Can you work these out from the drawing? Everything is in mm from the part's minimum corner. Give positions to 0.01 mm unless a question says otherwise; leave off trailing zeros. Write each loop counter-clockwise with the first axis right and the second up, starting at its lowest first coordinate (ties: lowest second). Pieces come first, ordered by that corner, then holes. Notation, with made-up numbers: (16, 7.5) - (38, 7.5) arc R18 ccw to (38, 26.5) - close; hole circle Ø4 at (-23.5, 9). An arc over 180 degrees is marked (long way). Use a Markdown table: item, result.
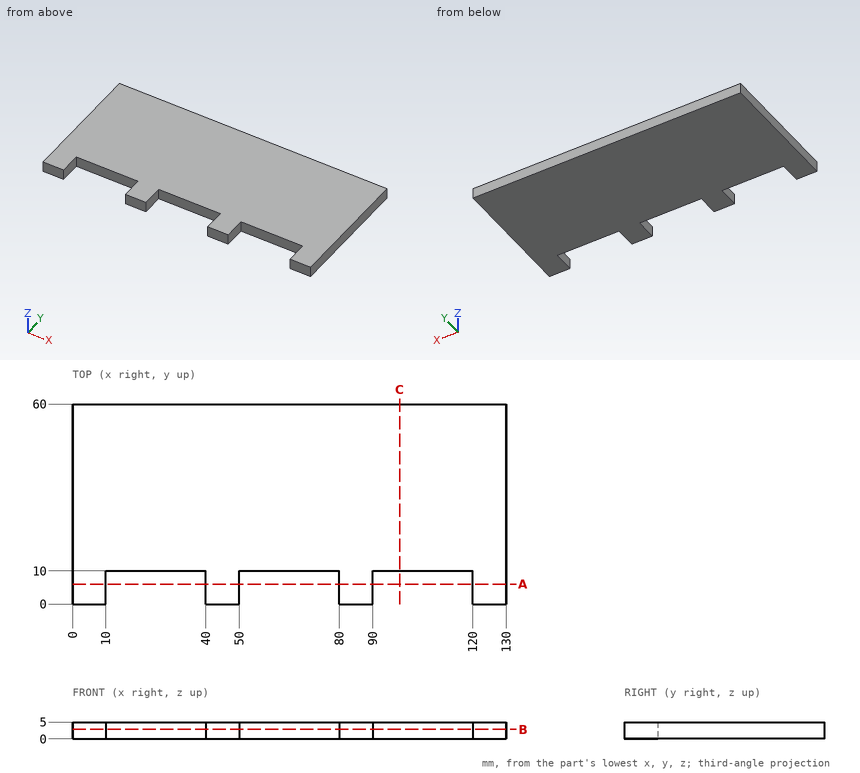
Item 1: If we section it at C-C, the plane x = 98: Write out the boundary of the cut face in (y, z), plus the area to 3 significant figures.
Values:
| item | result |
|---|---|
| outline | (10, 0) - (60, 0) - (60, 5) - (10, 5) - close |
| area | 250 mm2 |
Item 2: I need wall thicknesses on line 1 along X through (y, z) = (6, 3.6); line 2 along Y through (x, z) = (119.5, 3.3). Which ranges of each line are inside material? Lowest first, please. Write a range as [from, to].
Values:
| item | result |
|---|---|
| line 1 | x = [0, 10], [40, 50], [80, 90], [120, 130] |
| line 2 | y = [10, 60] |
Item 3: Will this pin go through, and if not, where does the flat tip stop? pin 1 Ø1.5 at (x, z) = (62.5, 2.5) entering from -Y.
Values:
| item | result |
|---|---|
| pin 1 | stops at y = 10 |
Item 4: If we section it at B-B, the plane z = 2.85: Write out the boundary of the cut face in (x, y).
Values:
| item | result |
|---|---|
| outline | (0, 0) - (10, 0) - (10, 10) - (40, 10) - (40, 0) - (50, 0) - (50, 10) - (80, 10) - (80, 0) - (90, 0) - (90, 10) - (120, 10) - (120, 0) - (130, 0) - (130, 60) - (0, 60) - close |
Item 5: If we section it at A-A, the plane y = 6: Write out the boundary of the cut face in (x, z), plus the area to 3 significant figures.
Values:
| item | result |
|---|---|
| outline | (0, 0) - (10, 0) - (10, 5) - (0, 5) - close; (40, 0) - (50, 0) - (50, 5) - (40, 5) - close; (80, 0) - (90, 0) - (90, 5) - (80, 5) - close; (120, 0) - (130, 0) - (130, 5) - (120, 5) - close |
| area | 200 mm2 |
